Source: CAD feature listing. Evaluate the final solid. Frame: model axes, mm. Coordinates: 2 decimals unless noted, no trailing zeros. Write each loop counter-clockwise with the first axis right and the second up, starting at its lowest first coordinate (ties: lowest second). Pieces come first, ordered by that corner, then holes. Notation, with made-up numbers: (61, 46.25) -> (119, 46.25) arc R18 cw to (119, 68.25) -> close; hole circle Ø4 at (54.25, -34). An arc over 180 degrees is marked (long way). One line per item, written item: value. Start each with the question number.
1. Section query B-B, the plane z = -80. Output: boundary loops of the cut face in (x, y).
2. Section query D-D, the plane y = 0.3. State how many separate pieces and enclosed holes the cut face has, and give its area (3 significant figures).
3. Section query A-A, the plane x = -17. Output: boundary loops of the cut face in (y, z), and give its area (3 significant figures).
4. Mould query, pull axis X, two halves, no side actions, for faces 1 (the flat face through (32.7, 0.99, 21.19)), 2 (the flat face through (23.526, 1.014, -87.302)), 3 (the cylindrical face through (-35.92, 0.99, -118.67)). Classes: released by +X, released by -X, zero draft, split by the parting line, or undercut.
5. Section query C-C, the plane z = 40. Output: boundary loops of the cut face in (x, y), and give its area (3 significant figures).
6. First-contact query: P1, Ø0.6, axis at y = 1, z = -16.5, coming from the -X side; P2, Ø2.5, axis at x = -34.5, z = -72, coming from the +Y side; P3, Ø1, axis at y = 0.5, z = -46.5, coming from the +X side; P4, Ø1, axis at y = 1.5, z = -87, coming from the -X side. Flat tips, straight axial feed; report the tip coordinate or a pass-through.
7. Line query: line 1 (X direction, y = 1.8, z = -102); line 2 (X direction, y = 1.25, z = 102); line 3 (Z direction, x = 18, y = 1.7). Output: solid intervals per line, ascending.
from build123d import *

# Parameters (mm, degrees)
SKETCH1_R           = 3
SKETCH1_R_2         = 1.65
BOSS_EXTRUDE1_DEPTH = 2
BOSS_EXTRUDE2_START = -2
SKETCH2_R           = 5.090936199
SKETCH2_R_2         = 1.65
BOSS_EXTRUDE2_DEPTH = 2
SKETCH3_R           = 1.65
CUT_EXTRUDE1_DEPTH  = 10
SKETCH4_R           = 1.75
CUT_EXTRUDE2_DEPTH  = 10


with BuildPart() as part:
    # Sketch1 → Boss-Extrude1 (new body)
    with BuildSketch(Plane(origin=(0, 0, 0), x_dir=(1, 0, 0), z_dir=(0, 1, 0))):
        with BuildLine():
            Line((37.525062814, 115), (37.525062814, 23.974506194))
            Line((37.525062814, 23.974506194), (28, 18.475208614))
            Line((28, 18.475208614), (28, -18.475208614))
            Line((28, -18.475208614), (37.525062814, -23.974506194))
            Line((37.525062814, -23.974506194), (37.525062814, -115))
            ThreePointArc((37.525062814, -115), (36.05174681, -118.544424535), (32.5, -120))
            Line((32.5, -120), (-32.5, -120))
            ThreePointArc((-32.5, -120), (-36.224769498, -118.363426816), (-37.5, -114.5))
            Line((-37.5, -114.5), (-37.5, -23.960036171))
            Line((-37.5, -23.960036171), (-28, -18.475208614))
            Line((-28, -18.475208614), (-28, 18.475208614))
            Line((-28, 18.475208614), (-37.5, 23.960036171))
            Line((-37.5, 23.960036171), (-37.5, 115.5))
            ThreePointArc((-37.5, 115.5), (-35.879164781, 118.708099244), (-32.525062814, 120))
            Line((-32.525062814, 120), (32.525062814, 120))
            ThreePointArc((32.525062814, 120), (36.06059672, 118.535533906), (37.525062814, 115))
        make_face()
        with Locations(Location((-27.497748671, 63.999999894, 0), (0, 0, 270))):
            Circle(SKETCH1_R, mode=Mode.SUBTRACT)
        with Locations(Location((-27.498874335, 51.999999947, 0), (0, 0, 270))):
            Circle(SKETCH1_R, mode=Mode.SUBTRACT)
        with Locations(Location((-27.5, 40, 0), (0, 0, 270))):
            Circle(SKETCH1_R, mode=Mode.SUBTRACT)
        with Locations(Location((27.5, 40, 0), (0, 0, 90))):
            Circle(SKETCH1_R, mode=Mode.SUBTRACT)
        with Locations(Location((27.498874335, 51.999999947, 0), (0, 0, 90))):
            Circle(SKETCH1_R, mode=Mode.SUBTRACT)
        with Locations(Location((27.497748671, 63.999999894, 0), (0, 0, 90))):
            Circle(SKETCH1_R, mode=Mode.SUBTRACT)
        with Locations(Location((27.497748671, -63.999999894, 0), (0, 0, 270))):
            Circle(SKETCH1_R, mode=Mode.SUBTRACT)
        with Locations(Location((27.498874335, -51.999999947, 0), (0, 0, 270))):
            Circle(SKETCH1_R, mode=Mode.SUBTRACT)
        with Locations(Location((27.5, -40, 0), (0, 0, 270))):
            Circle(SKETCH1_R, mode=Mode.SUBTRACT)
        with Locations(Location((-27.5, -40, 0), (0, 0, 90))):
            Circle(SKETCH1_R, mode=Mode.SUBTRACT)
        with Locations(Location((-27.498874335, -51.999999947, 0), (0, 0, 90))):
            Circle(SKETCH1_R, mode=Mode.SUBTRACT)
        with Locations(Location((-27.497748671, -63.999999894, 0), (0, 0, 90))):
            Circle(SKETCH1_R, mode=Mode.SUBTRACT)
        with Locations(Location((-34.497748671, 71.999999894, 0), (0, 0, 270))):
            Circle(SKETCH1_R_2, mode=Mode.SUBTRACT)
        with Locations(Location((34.497748671, 71.999999894, 0), (0, 0, 90))):
            Circle(SKETCH1_R_2, mode=Mode.SUBTRACT)
        with Locations(Location((34.497748671, -71.999999894, 0), (0, 0, 270))):
            Circle(SKETCH1_R_2, mode=Mode.SUBTRACT)
        with Locations(Location((-34.497748671, -71.999999894, 0), (0, 0, 90))):
            Circle(SKETCH1_R_2, mode=Mode.SUBTRACT)
    extrude(amount=BOSS_EXTRUDE1_DEPTH)

    # Sketch2 → Boss-Extrude2 (add)
    # profile 1 of 4: a face of its own
    with BuildSketch(Plane(origin=(0, 2, 0), x_dir=(1, 0, 0), z_dir=(0, 1, 0)).offset(BOSS_EXTRUDE2_START)):
        with Locations((-34.497748671, 71.999999894)):
            Circle(SKETCH2_R)
        with Locations(Location((-34.497748671, 71.999999894, 0), (0, 0, 270))):
            Circle(SKETCH2_R_2, mode=Mode.SUBTRACT)
    # profile 2 of 4: a face of its own
    with BuildSketch(Plane(origin=(0, 2, 0), x_dir=(1, 0, 0), z_dir=(0, 1, 0)).offset(BOSS_EXTRUDE2_START)):
        with Locations((34.497748671, 71.999999894)):
            Circle(SKETCH2_R)
        with Locations(Location((34.497748671, 71.999999894, 0), (0, 0, 90))):
            Circle(SKETCH2_R_2, mode=Mode.SUBTRACT)
    # profile 3 of 4: a face of its own
    with BuildSketch(Plane(origin=(0, 2, 0), x_dir=(1, 0, 0), z_dir=(0, 1, 0)).offset(BOSS_EXTRUDE2_START)):
        with Locations((34.497748671, -71.999999894)):
            Circle(SKETCH2_R)
        with Locations(Location((34.497748671, -71.999999894, 0), (0, 0, 270))):
            Circle(SKETCH2_R_2, mode=Mode.SUBTRACT)
    # profile 4 of 4: a face of its own
    with BuildSketch(Plane(origin=(0, 2, 0), x_dir=(1, 0, 0), z_dir=(0, 1, 0)).offset(BOSS_EXTRUDE2_START)):
        with Locations((-34.497748671, -71.999999894)):
            Circle(SKETCH2_R)
        with Locations(Location((-34.497748671, -71.999999894, 0), (0, 0, 90))):
            Circle(SKETCH2_R_2, mode=Mode.SUBTRACT)
    extrude(amount=BOSS_EXTRUDE2_DEPTH)

    # Sketch3 → Cut-Extrude1 (cut)
    with BuildSketch(Plane(origin=(0, 2, 0), x_dir=(1, 0, 0), z_dir=(0, 1, 0))):
        with Locations(Location((-32.5, 114, 0), (0, 0, 270))):
            Circle(SKETCH3_R)
        with Locations(Location((-32.5, 102, 0), (0, 0, 270))):
            Circle(SKETCH3_R)
        with Locations(Location((-32.5, 86, 0), (0, 0, 270))):
            Circle(SKETCH3_R)
        with Locations(Location((-32.5, 28, 0), (0, 0, 270))):
            Circle(SKETCH3_R)
        with Locations(Location((32.5, 28, 0), (0, 0, 90))):
            Circle(SKETCH3_R)
        with Locations(Location((32.5, 86, 0), (0, 0, 90))):
            Circle(SKETCH3_R)
        with Locations(Location((32.5, 102, 0), (0, 0, 90))):
            Circle(SKETCH3_R)
        with Locations(Location((32.5, 114, 0), (0, 0, 90))):
            Circle(SKETCH3_R)
        with Locations(Location((32.5, -114, 0), (0, 0, 270))):
            Circle(SKETCH3_R)
        with Locations(Location((32.5, -102, 0), (0, 0, 270))):
            Circle(SKETCH3_R)
        with Locations(Location((32.5, -86, 0), (0, 0, 270))):
            Circle(SKETCH3_R)
        with Locations(Location((32.5, -28, 0), (0, 0, 270))):
            Circle(SKETCH3_R)
        with Locations(Location((0, -96.35, 0), (0, 0, 270))):
            Circle(SKETCH3_R)
        with Locations(Location((-32.5, -28, 0), (0, 0, 90))):
            Circle(SKETCH3_R)
        with Locations(Location((-32.5, -86, 0), (0, 0, 90))):
            Circle(SKETCH3_R)
        with Locations(Location((-32.5, -102, 0), (0, 0, 90))):
            Circle(SKETCH3_R)
        with Locations(Location((-32.5, -114, 0), (0, 0, 90))):
            Circle(SKETCH3_R)
        Polygon((0, 82.909485966), (-8.660254038, 77.909485966), (-8.660254038, 67.909485966), (0, 62.909485966), (8.660254038, 67.909485966), (8.660254038, 77.909485966), align=None)
        Polygon((0, 110.909485966), (-8.660254038, 105.909485966), (-8.660254038, 95.909485966), (0, 90.909485966), (8.660254038, 95.909485966), (8.660254038, 105.909485966), align=None)
        Polygon((0, 54.909485966), (-8.660254038, 49.909485966), (-8.660254038, 39.909485966), (0, 34.909485966), (8.660254038, 39.909485966), (8.660254038, 49.909485966), align=None)
        Polygon((0, 26.909485966), (-8.660254038, 21.909485966), (-8.660254038, 11.909485966), (0, 6.909485966), (8.660254038, 11.909485966), (8.660254038, 21.909485966), align=None)
        Polygon((0, -1.090514034), (-8.660254038, -6.090514034), (-8.660254038, -16.090514034), (0, -21.090514034), (8.660254038, -16.090514034), (8.660254038, -6.090514034), align=None)
        Polygon((0, -29.090514034), (-8.660254038, -34.090514034), (-8.660254038, -44.090514034), (0, -49.090514034), (8.660254038, -44.090514034), (8.660254038, -34.090514034), align=None)
        Polygon((0, -57.090514034), (-8.660254038, -62.090514034), (-8.660254038, -72.090514034), (0, -77.090514034), (8.660254038, -72.090514034), (8.660254038, -62.090514034), align=None)
        with BuildLine():
            Line((-10.125189832, 116.65), (-3.874810168, 116.65))
            ThreePointArc((-3.874810168, 116.65), (-2.224810168, 115), (-3.874810168, 113.35))
            Line((-3.874810168, 113.35), (-10.125189832, 113.35))
            ThreePointArc((-10.125189832, 113.35), (-11.775189832, 115), (-10.125189832, 116.65))
        make_face()
        with BuildLine():
            Line((10.125189832, 116.65), (3.874810168, 116.65))
            ThreePointArc((3.874810168, 116.65), (2.224810168, 115), (3.874810168, 113.35))
            Line((3.874810168, 113.35), (10.125189832, 113.35))
            ThreePointArc((10.125189832, 113.35), (11.775189832, 115), (10.125189832, 116.65))
        make_face()
        with BuildLine():
            Line((10.125189832, -116.65), (3.874810168, -116.65))
            ThreePointArc((3.874810168, -116.65), (2.224810168, -115), (3.874810168, -113.35))
            Line((3.874810168, -113.35), (10.125189832, -113.35))
            ThreePointArc((10.125189832, -113.35), (11.775189832, -115), (10.125189832, -116.65))
        make_face()
        with BuildLine():
            Line((-10.125189832, -116.65), (-3.874810168, -116.65))
            ThreePointArc((-3.874810168, -116.65), (-2.224810168, -115), (-3.874810168, -113.35))
            Line((-3.874810168, -113.35), (-10.125189832, -113.35))
            ThreePointArc((-10.125189832, -113.35), (-11.775189832, -115), (-10.125189832, -116.65))
        make_face()
        Polygon((12.669872981, 83.5), (8.339745962, 91), (12.669872981, 98.5), (21.330127019, 98.5), (25.660254038, 91), (21.330127019, 83.5), align=None)
        Polygon((-8.339745962, 91), (-12.669872981, 98.5), (-21.330127019, 98.5), (-25.660254038, 91), (-21.330127019, 83.5), (-12.669872981, 83.5), align=None)
        Polygon((21.330127019, -83.5), (12.669872981, -83.5), (8.339745962, -91), (12.669872981, -98.5), (21.330127019, -98.5), (25.660254038, -91), align=None)
        Polygon((-12.669872981, -83.5), (-8.339745962, -91), (-12.669872981, -98.5), (-21.330127019, -98.5), (-25.660254038, -91), (-21.330127019, -83.5), align=None)
    extrude(amount=-CUT_EXTRUDE1_DEPTH, mode=Mode.SUBTRACT)

    # Sketch4 → Cut-Extrude2 (cut)
    with BuildSketch(Plane(origin=(0, 2, 0), x_dir=(1, 0, 0), z_dir=(0, 1, 0))):
        with Locations(Location((-21, -78.35, 0), (0, 0, 270))):
            Circle(SKETCH4_R)
        with Locations(Location((21, -78.35, 0), (0, 0, 270))):
            Circle(SKETCH4_R)
        with Locations(Location((-21, 0.65, 0), (0, 0, 270))):
            Circle(SKETCH4_R)
        with Locations(Location((21, 0.65, 0), (0, 0, 270))):
            Circle(SKETCH4_R)
    extrude(amount=-CUT_EXTRUDE2_DEPTH, mode=Mode.SUBTRACT)


solid = part.part
Computed values:
1. outline: (-37.5, 0) -> (-5.04, 0) -> (-5.04, 2) -> (-37.5, 2) -> close; (5.04, 0) -> (37.53, 0) -> (37.53, 2) -> (5.04, 2) -> close
2. separate pieces: 1
2. enclosed holes: 52
2. area: 14,000 mm²
3. outline: (0, -120) -> (2, -120) -> (2, -98.5) -> (0, -98.5) -> close; (0, -83.5) -> (2, -83.5) -> (2, 83.5) -> (0, 83.5) -> close; (0, 98.5) -> (2, 98.5) -> (2, 120) -> (0, 120) -> close
3. area: 420 mm²
4. face 1: released by +X
4. face 2: undercut
4. face 3: released by -X
5. outline: (-37.5, 0) -> (-30.5, 0) -> (-30.5, 2) -> (-37.5, 2) -> close; (-24.5, 0) -> (-8.66, 0) -> (-8.66, 2) -> (-24.5, 2) -> close; (8.66, 0) -> (24.5, 0) -> (24.5, 2) -> (8.66, 2) -> close; (30.5, 0) -> (37.53, 0) -> (37.53, 2) -> (30.5, 2) -> close
5. area: 91.4 mm²
6. P1: stops at x = -28
6. P2: passes through
6. P3: stops at x = 37.53
6. P4: stops at x = -37.5
7. line 1: x = -37.5 to -34.15, -30.85 to -8.66, 8.66 to 30.85, 34.15 to 37.53
7. line 2: x = -37.5 to -34.15, -30.85 to 30.85, 34.15 to 37.53
7. line 3: z = -120 to -98.5, -83.5 to 83.5, 98.5 to 120
